Part model, mm, in its own coordinate system. A direction names the side the tool comes from. Give positions to 0.01 mm unless a question says otherwise; leave off trailing zeros. Loops run counter-clockwise (first coordinate to the right, second up) from the corner with the lowest first, then second, coordinate; pieces in that order, holes last. Notation, with made-up numbers: (48.5, 43.25) -> (69.5, 43.25) arc R24 ccw to (69.5, 78.25) -> close; hole circle Ø10 at (53.25, 23). An arc over 180 degrees is marked (long way). Write item = value, one per line.
from build123d import *

# Parameters (mm, degrees)
BOSS_EXTRUDE1_DEPTH     = 4.5
CUT_EXTRUDE1_DEPTH      = 10
CUT_EXTRUDE2_DEPTH      = 5.5
CUT_EXTRUDE2_DEPTH_BACK = 5.5
FILLET1_R               = 2.5
FILLET2_R               = 0.75


with BuildPart() as part:
    # Sketch2 → Boss-Extrude1 (new body, symmetric)
    with BuildSketch(Plane(origin=(0, 0, 0), x_dir=(0, 0, -1), z_dir=(1, 0, 0))):
        Polygon((2, -9), (2, -10.6), (-6, -10.6), (-6, -13.6), (5, -13.6), (5, -9), (5, 9), (-5, 9), (-5, -9), align=None)
    extrude(amount=BOSS_EXTRUDE1_DEPTH, both=True)

    # Sketch3 → Cut-Extrude1 (cut)
    with BuildSketch(Plane.XY.offset(5)):
        Polygon((-3, 6.5), (-3, -6.5), (3, -6.5), (3, 6.5), (3, 9), (-3, 9), align=None)
    extrude(amount=-CUT_EXTRUDE1_DEPTH, mode=Mode.SUBTRACT)

    # Sketch4 → Cut-Extrude2 (cut, two sides)
    with BuildSketch(Plane(origin=(0, 0, 0), x_dir=(0, 0, -1), z_dir=(1, 0, 0))) as cut_extrude2_sk:
        Polygon((0.775352078, 4.225), (-1, 7.3), (-2.775352078, 4.225), align=None)
        Polygon((0.775352078, -2.275), (-1, 0.8), (-2.775352078, -2.275), align=None)
    extrude(amount=CUT_EXTRUDE2_DEPTH, mode=Mode.SUBTRACT)
    extrude(cut_extrude2_sk.sketch, amount=-CUT_EXTRUDE2_DEPTH_BACK, mode=Mode.SUBTRACT)

    # Fillet1
    fillet1_edges = [part.edges().sort_by_distance(p)[0] for p in [
        (0, -13.6, -5),
        (3.75, 9, 5),
        (3.75, 9, -5),
        (4.5, -12.1, 6),
        (-3.75, 9, 5),
        (-3.75, 9, -5),
        (-4.5, -12.1, 6),
    ]]
    fillet(fillet1_edges, radius=FILLET1_R)

    # Fillet2
    fillet2_edges = [part.edges().sort_by_distance(p)[0] for p in [
        (0, -10.6, -2),
        (0, -9, -2),
    ]]
    fillet(fillet2_edges, radius=FILLET2_R)


solid = part.part
1) Slice it at D-D, the plane z = 4.75. List the corners of the cut face in (x, y).
Resolved:
outline = (-4.5, -9) -> (4.5, -9) -> (4.5, 7.59) -> (3, 7.59) -> (3, -6.5) -> (-3, -6.5) -> (-3, 7.59) -> (-4.5, 7.59) -> close; (-4.17, -13.6) -> (4.17, -13.6) -> (4.17, -10.6) -> (-4.17, -10.6) -> close
2) Slice it at A-A, the plane y = 2. List the corners of the cut face in (x, z), and give its area (3 significant figures).
Resolved:
outline = (-4.5, -5) -> (-3, -5) -> (-3, 5) -> (-4.5, 5) -> close; (3, -5) -> (4.5, -5) -> (4.5, 5) -> (3, 5) -> close
area = 30.0 mm²
3) Pull direction Y, two halves, no side cores. Call faces 1 (the face through (4, -4, -5)), 2 (the face through (-4, 9, 0)), 3 (the face through (-4, 4.225, 1)): pulls with the +Y half, pulls with the -Y half, needs draft (parallel to the pull), parting line crosses it, or undercut.
Resolved:
face_1 = needs draft
face_2 = pulls with the +Y half
face_3 = undercut
4) Slice it at B-B, the plane x = 3.5. List the corners of the cut face in (y, z) (3 decimals), and give its area (3 significant figures).
Resolved:
outline = (-13.6, -2.5) arc R2.5 ccw to (-11.1, -5) -> (6.5, -5) arc R2.5 ccw to (9, -2.5) -> (9, 2.5) arc R2.5 ccw to (6.5, 5) -> (-9, 5) -> (-9, -1.25) arc R0.75 cw to (-9.75, -2) -> (-9.85, -2) arc R0.75 cw to (-10.6, -1.25) -> (-10.6, 5.5) -> (-13.6, 5.5) -> close; hole (-2.275, -0.775) -> (0.8, 1) -> (-2.275, 2.775) -> close; hole (4.225, -0.775) -> (7.3, 1) -> (4.225, 2.775) -> close
area = 202 mm²
5) Slice it at C-C, the plane z = -0.25. List the corners of the cut face in (x, y) (3 decimals), and give its area (3 significant figures).
Resolved:
outline = (-4.5, -13.6) -> (4.5, -13.6) -> (4.5, -10.6) -> (-4.5, -10.6) -> close; (-4.5, -9) -> (4.5, -9) -> (4.5, -2.275) -> (3, -2.275) -> (3, -6.5) -> (-3, -6.5) -> (-3, -2.275) -> (-4.5, -2.275) -> close; (-4.5, -1.365) -> (-3, -1.365) -> (-3, 4.225) -> (-4.5, 4.225) -> close; (-4.5, 5.135) -> (-3, 5.135) -> (-3, 9) -> (-4.5, 9) -> close; (3, -1.365) -> (4.5, -1.365) -> (4.5, 4.225) -> (3, 4.225) -> close; (3, 5.135) -> (4.5, 5.135) -> (4.5, 9) -> (3, 9) -> close
area = 90.5 mm²
6) Which spindle directions (+Z, -Z, +X, -X, +Y, -Y) get a long thin tool onto all of the face, cutting with end or side? Do faces 4 (the face through (4, -12, 5)), 5 (the face through (4, -3, 5)), 6 (the face through (3, 1, 0)), 7 (the face through (3.74, 5.74, 0.1)). Say none if no direction does.
Resolved:
face_4 = +Z, +X, -Y
face_5 = +Z, +X, -X, +Y
face_6 = +Z, -Z, +Y
face_7 = +X, -X
7) Drill centre lines: line 1 along X through (y, z) = (-6, -3.5); line 2 along Y through (x, z) = (-1.5, -1.25); line 3 along Y through (x, z) = (-4, -0.5) (3 decimals). Where is each one in solid material? Low to high. Write a range as [from, to].
Resolved:
line_1 = [-4.5, -3], [3, 4.5]
line_2 = [-13.6, -10.6], [-9, -6.5]
line_3 = [-13.6, -10.6], [-9, -2.275], [-1.798, 4.225], [4.702, 9]
8) Drop flat-ended pins along their axis: P1, Ø4, axis at x = 0, y = -9.5, coming from the +Z side; P2, Ø1, axis at x = 3.5, y = 5, coming from the +Z side; P3, Ø3, axis at x = 0.5, z = 1.5, coming from the +Y side. Give the stop position or say it passes through.
Resolved:
P1 = 6
P2 = 5
P3 = -6.5
